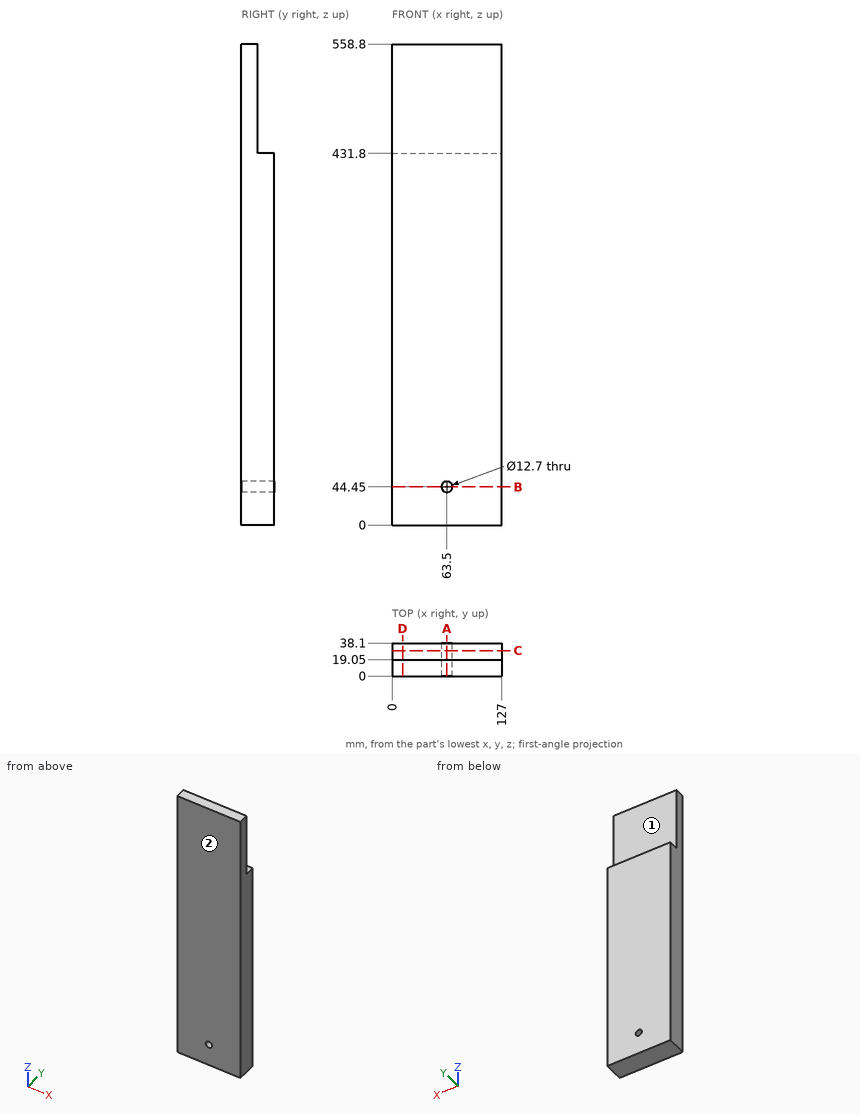
Can you work these out from the drawing? Everything is in mm from the part's minimum corner. Coordinates: 2 decimals unless noted, no trailing zeros. Loops run counter-clockwise (first coordinate to the right, second up) from the corner with the lowest first, then second, coordinate; pieces in that order, holes last.
1. Imagine slicing it at B-B, the plane z = 44.45. Please give me the cut outline in (x, y).
2. Imagine slicing it at C-C, the plane y = 29.5. Please give me the cut outline in (x, z), and give its area (3 significant figures).
3. For P1, Ø15, axis at x = 60.5, y = 27, coming from the +Z side, with a flat end and sliding along its axis, tell me the tip position at first contact or that it passes through.
4. I need wall thicknesses on L1, parallel to Z at x = 63.5, y = 23.5; L2, parallel to X at y = 24, z = 44.45; L3, parallel to Z at x = 63, y = 10. Which ranges of each line are inside material? Lowest first, please.
5. Imagine slicing it at A-A, the plane x = 63.5. Please give me the cut outline in (y, z), and give its area (3 significant figures).
6. Imagine slicing it at D-D, the plane x = 12. Please give me the cut outline in (y, z).
7. If we mould it in two halves opening along Y, with no side actions, what happens to the marked faces 1 and 2? For each: pulls with the +Y half, pulls with the -Y half, needs draft (parallel to the pull), parting line crosses it, or undercut.
Taken from the geometry:
1. outline: (0, 0) - (57.15, 0) - (57.15, 38.1) - (0, 38.1) - close; (69.85, 0) - (127, 0) - (127, 38.1) - (69.85, 38.1) - close
2. outline: (0, 0) - (127, 0) - (127, 431.8) - (0, 431.8) - close; hole circle Ø12.7 at (63.5, 44.45)
2. area: 54,700 mm2
3. P1: stops at z = 431.8
4. L1: z = 0 to 38.1, 50.8 to 431.8
4. L2: x = 0 to 57.15, 69.85 to 127
4. L3: z = 0 to 38.12, 50.78 to 558.8
5. outline: (0, 0) - (38.1, 0) - (38.1, 38.1) - (0, 38.1) - close; (0, 50.8) - (38.1, 50.8) - (38.1, 431.8) - (19.05, 431.8) - (19.05, 558.8) - (0, 558.8) - close
5. area: 18,400 mm2
6. outline: (0, 0) - (38.1, 0) - (38.1, 431.8) - (19.05, 431.8) - (19.05, 558.8) - (0, 558.8) - close
7. face 1: pulls with the +Y half
7. face 2: pulls with the -Y half
